Read the model definition and answer for the solid it produces. Units are mm, in the model's axes. A direction names the side the tool comes from. Give positions to 0.01 mm unless a question says otherwise; leave off trailing zeros. Order: outer loops, then holes, each group sorted by start corner. A loop starts at its lowest first (then second) coordinate and runs counter-clockwise, first axis right, second up.
Autodesk Inventor part; units mm, degrees
ref_plane "YZ Plane" through (0, 0, 0) normal (1, 0, 0) x (0, 1, 0)
ref_plane "XZ Plane" through (0, 0, 0) normal (0, 1, 0) x (-1, 0, 0)
ref_plane "XY Plane" through (0, 0, 0) normal (0, 0, 1) x (1, 0, 0)
sketch "Skizze1" plane through (0, 0, 0) normal (0, 0, 1) x (1, 0, 0)
  circle A0 centre (0, 0) radius 10.5
  circle A1 centre (0, 0) radius 12.55
  dimension "d0" = 25.1
  dimension "d1" = 2.05
extrude "Extrusion1" add sketch "Skizze1" along normal blind 274
sketch "Skizze2" plane through (0, 0, 274) normal (0, 0, 1) x (1, 0, 0)
  circle A0 centre (0, 0) radius 12.55
  circle A1 centre (0, 0) radius 12.25
  dimension "d4" = 24.5
extrude "Extrusion2" cut sketch "Skizze2" against normal through all
sketch "Skizze3" plane through (0, 0, 0) normal (0, 0, -1) x (-1, 0, 0)
  circle A0 centre (0, 0) radius 12.25
  circle A1 centre (0, 0) radius 10.5
  circle A2 centre (0, 0) radius 12.5
  dimension "d7" = 25
extrude "Extrusion3" add sketch "Skizze3" against normal blind 9 contours A2
sketch "Skizze4" plane through (0, 0, 274) normal (0, 0, 1) x (1, 0, 0)
  circle A0 centre (0, 0) radius 12.25
  circle A1 centre (0, 0) radius 10.5
  circle A2 centre (0, 0) radius 11.5
  dimension "d10" = 23
extrude "Extrusion4" cut sketch "Skizze4" against normal blind 50 contours A0
sketch "Skizze5" plane through (0, 0, 0) normal (0, 1, 0) x (-1, 0, 0)
  line L0 (-12.5, 9) -> (12.5, 9)
  line L1 (12.5, 0) -> (-12.5, 0)
  line L2 (12.25, 9) -> (-12.25, 9)
  line L3 (12.5, 0) -> (12.5, 9)
  line L4 (10.5, 0) -> (10.5, 274)
  line L5 (12.25, 224) -> (12.25, 9)
  line L6 (12.5, 9) -> (11.75, 9)
  line L7 (11.75, 9) -> (11.75, 7)
  line L8 (11.75, 7) -> (12.5, 7)
  line L9 (12.5, 7) -> (12.5, 9)
  line L10 (17.5, 0) -> (-17.5, 0)
  line L11 (0, -54.8) -> (0, 328.8)
  point P0 (0, 0)
  point P1 (-9.75, 200)
  point P2 (9.75, 200)
  dimension "d13" = 2
  dimension "d14" = 23.5
revolve "Umdrehung1" cut sketch "Skizze5" angle 360 about axis through (0, 0, -10) along (0, 0, 1) contours L0 L3 L8 L7
chamfer "Fase1" distance 0.75 angle 45 1 edges at (12.5, 0, 7)
thread "Gewinde3"
fillet "Rundung1" radius 0.5 1 edges at (-11.5, 0, 224)
properties part number "13_0204_025"
1) A tool of negligible diameter and unlimited length cuts with its end or side. For faces 1 (the face through (-1.5, 11.4, 249.6)), 2 (the face through (-11.207, 3.529, 7.986)), 3 (the face through (-11.923, 3.755, 3.081)), from which of +Z, -Z, +X, -X, +Y, -Y can it reach the whole face along a straight path? Write none if from no direction.
Final values:
face 1: +Z
face 2: none
face 3: +Z, -Z
2) The part is cut by section D-D on z = 240.5. Determine the outline of the cut face in (x, y), and give its area (3 significant figures).
Final values:
outline: circle Ø23 at (0, 0); hole circle Ø21 at (0, 0)
area: 69.1 mm2
3) The part is cut by section C-C on z = 64. Determine the outline of the cut face in (x, y), and give its area (3 significant figures).
Final values:
outline: circle Ø24.5 at (0, 0); hole circle Ø21 at (0, 0)
area: 125 mm2
4) Consider L1, parallel to Y at x = 1, z = 215.5; L2, parallel to X at y = 0.5, z = 189; L3, parallel to Y at x = 1.25, z = 82. Determine where each line is inside the solid, lowest interval first.
Final values:
L1: y = -12.21 to -10.45, 10.45 to 12.21
L2: x = -12.24 to -10.49, 10.49 to 12.24
L3: y = -12.19 to -10.43, 10.43 to 12.19
5) Given pin 1 (3 mm diameter, centred on y = 2.5, z = 51, fed in from -X); pin 2 (3 mm diameter, centred on x = 9.5, z = 48, fed in from +Y); pin 3 (3 mm diameter, centred on x = 1.5, z = 141.5, fed in from +Y), each flat-ended and moving along its own axis, determine where each tip first touches the part or whether it passes through.
Final values:
pin 1: stops at x = -12.21
pin 2: stops at y = 9.28
pin 3: stops at y = 12.25
6) For a pull along X with two mould halves and no side action, classify faces 4 (the face through (6.586, 10.329, 118.005)), 5 (the face through (10, -3.2, 135.1)), 6 (the face through (-12, 1, 9)) as released by +X, released by -X, zero draft, split by the parting line, or undercut.
Final values:
face 4: split by the parting line
face 5: undercut
face 6: zero draft
